Part model, mm, in its own coordinate system. Face numbers are marked on the shaded views. A direction names the side the tool comes from. Give positions to 0.01 mm unless a question says otherwise; leave off trailing zeros. Order: outer loops, then holes, each group sorted by start corner. A loop starts at its lowest first (then second) coordinate and runs counter-clockwise, first axis right, second up. Notation, with made-up numbers: (66.5, 72.5) -> (110.5, 72.5) arc R27 ccw to (110.5, 98.5) -> close; hole circle Ø2 at (12.25, 79.25). An arc over 180 degrees is marked (long way). Write item = value, one per line. Start each with the question number.
(1) Probe line 1 along X through (y, z) = (9, 15); line 2 along Z through (x, y) = (-42, 20); line 3 along Z through (x, y) = (-21, 12). List the from-to ranges inside material, lowest first. Write a range as from..to.
(2) Saw through at A-A, the plane z = 31.5. List the corners of the cut face in (x, y).
(3) Flat gauge pins, fed straight in: pin 1 (15 mm diameter, centred on y = 15, z = 27, fed in from +X); pin 2 (24 mm diameter, centred on x = -41.5, y = 16.5, fed in from +Z); pin 3 (8 mm diameter, centred on x = -69, y = -2, fed in from +Z). Where does each tip first touch, or does it go through?
(4) Saw through at B-B, the plane x = -87.5. List the corners of the cut face in (y, z).
(5) Saw through at D-D, the plane z = 47. List the corners of the cut face in (x, y), then the cut area to 3 significant figures.
(6) Which spindle directions (+Z, -Z, +X, -X, +Y, -Y) get a long thin tool onto all of the face, cutting with end or side? Do the marked faces 1 and 2. Say none if no direction does.
(7) Two-plate mould, pull along X, no slides. Class the marked faces 3, 4 and 5: pulls with the +X half, pulls with the -X half, needs draft (parallel to the pull), parting line crosses it, or undercut.
(8) Saw through at C-C, the plane y = 11.5. List the corners of the cut face in (x, z).
from build123d import *

# Parameters (mm, degrees)
F0_W     = 63.5
F0_H     = 76.2
F1_DEPTH = 101.6
F3_W     = 50.8
F3_H     = 38.1
F4_DEPTH = 63.501
F5_DEPTH = 101.601


with BuildPart() as f1:
    # F0 (on Right) → F1 (new body)
    with BuildSketch(Plane.YZ):
        with Locations((1.986064, 14.267234)):
            Rectangle(F0_W, F0_H)
    extrude(amount=-F1_DEPTH)

    # F3 (on face) → F4 (cut, through all)
    with BuildSketch(Plane.XZ.offset(29.763936)):
        with Locations((-50.8, 33.317234)):
            Rectangle(F3_W, F3_H)
    extrude(amount=-F4_DEPTH, mode=Mode.SUBTRACT)

    # F2 (on face) → F5 (cut, through all)
    with BuildSketch(Plane.YZ):
        with BuildLine():
            ThreePointArc((-29.763936, 1.567234), (6.157089, 16.446209), (21.036064, 52.367234))
            Line((21.036064, 52.367234), (-29.763936, 52.367234))
            Line((-29.763936, 52.367234), (-29.763936, 1.567234))
        make_face()
        with BuildLine():
            Line((-29.763936, 52.367234), (21.036064, 52.367234))
            ThreePointArc((21.036064, 52.367234), (-65.68496, 88.288258), (-29.763936, 1.567234))
            Line((-29.763936, 1.567234), (-29.763936, 52.367234))
        make_face()
    extrude(amount=-F5_DEPTH, mode=Mode.SUBTRACT)


solid = f1.part
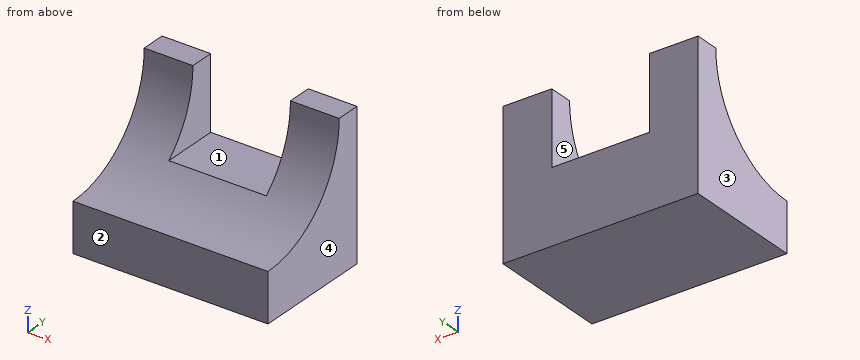
Results list:
q1.line_1 = -101.6..-76.2, -25.4..0
q1.line_2 = -23.83..14.27
q1.line_3 = -23.83..23.45
q2.outline = (-101.6, 16.55) -> (-76.2, 16.55) -> (-76.2, 33.74) -> (-101.6, 33.74) -> close; (-25.4, 16.55) -> (0, 16.55) -> (0, 33.74) -> (-25.4, 33.74) -> close
q3.pin_1 = 0
q3.pin_2 = 14.27
q3.pin_3 = 12.72
q4.outline = (-29.76, -23.83) -> (33.74, -23.83) -> (33.74, 52.37) -> (21.04, 52.37) arc R50.8 cw to (-29.76, 1.57) -> close
q5.outline = (-101.6, 20.75) -> (-76.2, 20.75) -> (-76.2, 33.74) -> (-101.6, 33.74) -> close; (-25.4, 20.75) -> (0, 20.75) -> (0, 33.74) -> (-25.4, 33.74) -> close
q5.area = 660 mm^2
q6.face_1 = +Z, +Y, -Y
q6.face_2 = +Z, -Z, +X, -X, -Y
q7.face_3 = pulls with the -X half
q7.face_4 = pulls with the +X half
q7.face_5 = undercut
q8.outline = (-101.6, -23.83) -> (0, -23.83) -> (0, 22.74) -> (-25.4, 22.74) -> (-25.4, 14.27) -> (-76.2, 14.27) -> (-76.2, 22.74) -> (-101.6, 22.74) -> close
